Source: CAD feature listing. Evaluate the final solid. Frame: model axes, mm. Round coordinates to 2 decimals unless told otherwise and drop trailing zeros. Loops run counter-clockwise (first coordinate to the right, second up) from the corner with the lowest first, then second, coordinate; pieces in that order, holes last. Notation, with made-up numbers: M 21,24.25 L 55,24.25 A35 cw 55,61.25 Z; hole C 60.25,19.25 d6. An arc over 180 degrees is marked long. Write each question's results on one line, items separated by ' | '. Start each with the question number.
1. Contact query for flat-ended pins moving along their axis: pin 1 Ø1.5 at (y, z) = (21.5, 5) entering from -X; pin 2 Ø1.5 at (x, z) = (10, 3) entering from -Y; pin 3 Ø4 at (x, z) = (-67.5, 5.5) entering from -Y. Output: stop coordinate, or through.
2. Section A-A on x = 8. Output: boundary loops of the cut face in (y, z).
3. Ray query, line 1 (Y direction, x = -25, z = 2.5); line 2 (X direction, y = -29.5, z = 2.5); line 3 (Y direction, x = 12, z = 5.25). Return the intervals inside material, ascending.
4. Section B-B on y = 10.5. Output: boundary loops of the cut face in (x, z).
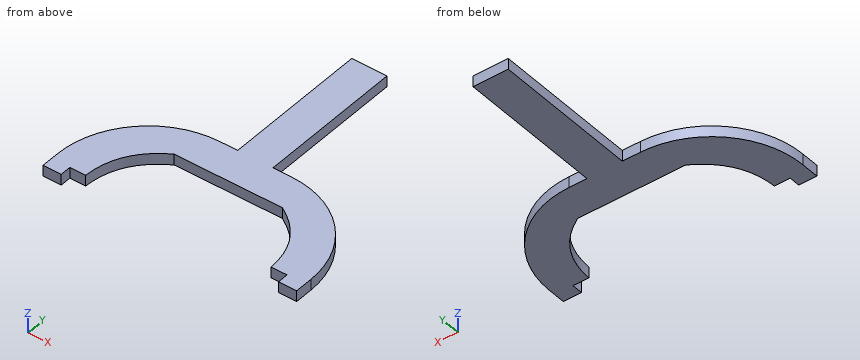
from build123d import *

# Parameters (mm, degrees)
BOSS_EXTRUDE1_DEPTH = 7.62
FILLET1_R           = 63.5
CUT_EXTRUDE1_DEPTH  = 155.990666284


with BuildPart() as part:
    # Sketch2 → Boss-Extrude1 (new body)
    with BuildSketch(Plane.XY):
        Polygon((12.315773934, -50.8), (88.515773934, -50.8), (88.515773934, -127), (75.815773934, -127), (75.815773934, -119.38), (37.715773934, -119.38), (37.715773934, -74.93), (-37.715773934, -74.93), (-37.715773934, -119.38), (-75.815773934, -119.38), (-75.815773934, -127), (-88.515773934, -127), (-88.515773934, -50.8), (-12.315773934, -50.8), (-12.315773934, 50.8), (12.315773934, 50.8), align=None)
    extrude(amount=BOSS_EXTRUDE1_DEPTH)

    # Fillet1
    fillet1_edges = [part.edges().sort_by_distance(p)[0] for p in [
        (88.515773934, -50.8, 3.81),
        (-88.515773934, -50.8, 3.81),
    ]]
    fillet(fillet1_edges, radius=FILLET1_R)

    # Sketch3 → Cut-Extrude1 (cut, through all)
    with BuildSketch(Plane.XY.offset(7.62)):
        with BuildLine():
            Line((-37.715773934, -74.93), (-37.715773934, -119.38))
            Line((-37.715773934, -119.38), (-64.735615427, -119.38))
            add(Edge.make_bspline(
                [(-64.735615427, -119.38), (-63.844183293, -90.073264765), (-37.715773934, -74.93)],
                knots=[0, 0, 0, 1, 1, 1], degree=2))
        make_face()
    cut_extrude1 = extrude(amount=-CUT_EXTRUDE1_DEPTH, mode=Mode.SUBTRACT)

    # Mirror1: Cut-Extrude1 across plane
    add(cut_extrude1.mirror(Plane.ZY), mode=Mode.SUBTRACT)


solid = part.part
Taken from the geometry:
1) pin 1: x = -12.32 | pin 2: y = -74.93 | pin 3: y = -119.38
2) outline: M -74.93,0 L 50.8,0 L 50.8,7.62 L -74.93,7.62 Z
3) line 1: -74.93 to -50.8 | line 2: -12.32 to 12.32 | line 3: -74.93 to 50.8
4) outline: M -12.32,0 L 12.32,0 L 12.32,7.62 L -12.32,7.62 Z
